Input: part model. Units: mm. Frame: model coordinates. Face numbers are marked on the shaded views. Coordinates: 2 decimals unless noted, no trailing zeros. Write each loop counter-clockwise with the first axis right and the second up, starting at its lowest first coordinate (ties: lowest second). Pieces come first, ordered by that corner, then holes.
1) Section query A-A (y = 0). Output: boundary loops of the cut face in (x, z), then the cut area to 3 significant figures.
2) Pin query (flat end, axial travel): pin 1 Ø4 at (x, z) = (10, 4.5) entering from +Y; pin 2 Ø3 at (x, z) = (10, 4.5) entering from -Y; pin 3 Ø18 at (y, z) = (0, 0) entering from +X; pin 4 Ø3 at (x, y) = (5.5, 12) entering from +Z. Return the tip coordinate at first contact, or that it passes through.
3) Line query: L1, parallel to Z at x = 7.25, y = 0; L2, parallel to Y at x = 8.5, z = -1.5. Output: solid intervals per line, ascending.
4) Section query C-C (x = 5). Output: boundary loops of the cut face in (y, z), then the cut area to 3 significant figures.
5) Draft query along Z for the marked faces 1, 2 and 3. Return one class per face: pulls with the +Z half, pulls with the -Z half, needs draft (parallel to the pull), parting line crosses it, or undercut.
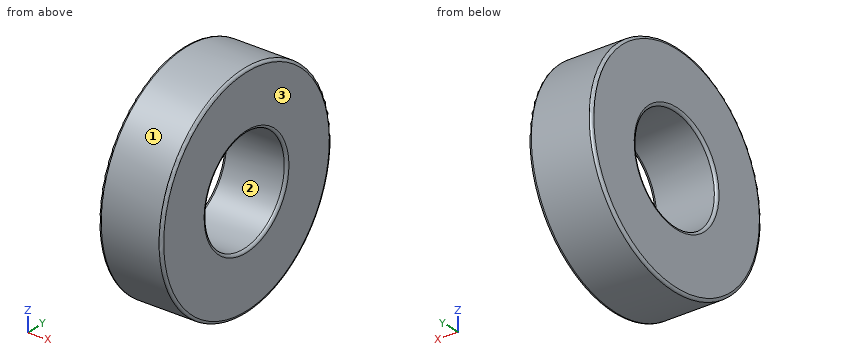
from build123d import *

# Parameters (mm, degrees)
F0_W = 12
F0_H = 11
F2_R = 0.5


with BuildPart() as f1:
    # F0 (on Front) → F1 (revolve)
    with BuildSketch(Plane.XZ):
        with Locations((6.26556, 15.5)):
            Rectangle(F0_W, F0_H)
    revolve(axis=Axis((2.772328, 0, 0), (1, 0, 0)))

    # F2
    f2_edges = [f1.edges().sort_by_distance(p)[0] for p in [
        (12.26556, 0, -21),
        (0.26556, 0, -21),
        (6.26556, 0, 21),
        (0.26556, 0, -10),
        (12.26556, 0, -10),
        (6.26556, 0, 10),
    ]]
    fillet(f2_edges, radius=F2_R)


solid = f1.part
Answer:
1. outline: (0.27, -20.5) arc R0.5 ccw to (0.77, -21) - (11.77, -21) arc R0.5 ccw to (12.27, -20.5) - (12.27, -10.5) arc R0.5 ccw to (11.77, -10) - (0.77, -10) arc R0.5 ccw to (0.27, -10.5) - close; (0.27, 10.5) arc R0.5 ccw to (0.77, 10) - (11.77, 10) arc R0.5 ccw to (12.27, 10.5) - (12.27, 20.5) arc R0.5 ccw to (11.77, 21) - (0.77, 21) arc R0.5 ccw to (0.27, 20.5) - close
1. area: 264 mm2
2. pin 1: stops at y = 20.85
2. pin 2: stops at y = -20.78
2. pin 3: passes through
2. pin 4: stops at z = 18.19
3. L1: z = -21 to -10, 10 to 21
3. L2: y = -20.95 to -9.89, 9.89 to 20.95
4. outline: circle Ø42 at (0, 0); hole circle Ø20 at (0, 0)
4. area: 1,070 mm2
5. face 1: parting line crosses it
5. face 2: undercut
5. face 3: needs draft
